Read the model definition and answer for the solid it produces. Units are mm, in the model's axes. Give positions to 0.01 mm unless a question says otherwise; leave off trailing zeros. Loops run counter-clockwise (first coordinate to the right, second up) from the corner with the lowest first, then second, coordinate; pieces in that order, holes last.
(1) Straight lines are drawn through the part: probe 1 along Y at (x, z) = (36.5, 6.25); probe 2 along Y at (x, z) = (0, 8.65); probe 3 along X at (y, z) = (-25, 2.2) (3 decimals). For each, find the intervals that lie inside material, in ascending order.
(2) Find section D-D, the plane z = 2.25. Write down the section's boundary in (x, y) (3 decimals), then the cut area to 3 significant figures.
(3) Find section B-B, the plane x = 0. Write down the section's boundary in (y, z) (3 decimals).
(4) This flat-tipped pin is pushed along its axis until it touches: P1, Ø3.5, axis at x = 2.5, y = 25, coming from the -Z side. Where does it stop, or does it pass through?
(5) Find section C-C, the plane y = -25. Write down the section's boundary in (x, z) (3 decimals).
(6) Find section A-A, the plane y = -36.5. Write down the section's boundary in (x, z), then the cut area to 3 significant figures.
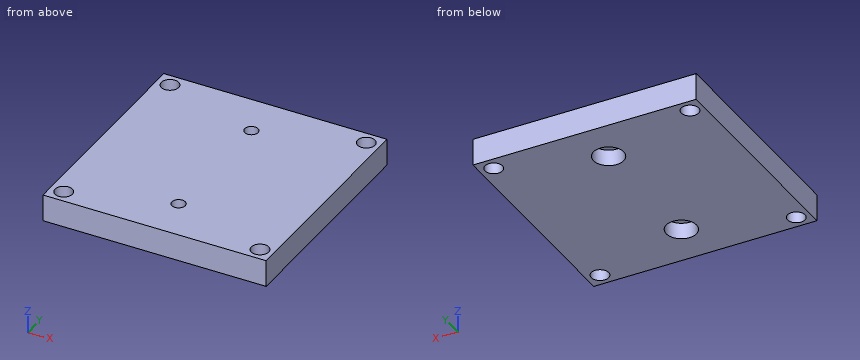
```python
from build123d import *

# Parameters (mm, degrees)
F0_W           = 83
F0_H           = 83
F1_DEPTH       = 10
F2_R           = 3.25
F3_DEPTH       = 10
F5_D           = 5
F5_DEPTH       = 15
F5_CBORE_D     = 11.25
F5_CBORE_DEPTH = 6
F5_TIP         = 1.5021515476


with BuildPart() as f1:
    # F0 (on Top) → F1 (new body)
    with BuildSketch(Plane.XY):
        Rectangle(F0_W, F0_H)
    extrude(amount=F1_DEPTH)

    # F2 (on face) → F3 (cut, through all)
    with BuildSketch(Plane.XY.offset(10)):
        with Locations((-36.5, 36.5)):
            Circle(F2_R)
        with Locations((-36.5, -36.5)):
            Circle(F2_R)
        with Locations((36.5, -36.5)):
            Circle(F2_R)
        with Locations((36.5, 36.5)):
            Circle(F2_R)
    extrude(amount=-F3_DEPTH, mode=Mode.SUBTRACT)

    # F5
    with Locations(Plane(origin=(0, 0, 0), x_dir=(1, 0, 0), z_dir=(0, 0, -1))):
        with Locations((0, -25), (0, 25)):
            CounterBoreHole(F5_D / 2, F5_CBORE_D / 2, F5_CBORE_DEPTH, depth=F5_DEPTH)
            with Locations((0, 0, -(F5_DEPTH + F5_TIP / 2))):  # 118° drill point
                Cone(0, F5_D / 2, F5_TIP, mode=Mode.SUBTRACT)


solid = f1.part
```
Entries:
1. probe 1: y = -41.5 to -39.75, -33.25 to 33.25, 39.75 to 41.5
1. probe 2: y = -41.5 to -27.5, -22.5 to 22.5, 27.5 to 41.5
1. probe 3: x = -41.5 to -5.625, 5.625 to 41.5
2. outline: (-41.5, -41.5) - (41.5, -41.5) - (41.5, 41.5) - (-41.5, 41.5) - close; hole circle Ø6.5 at (-36.5, -36.5); hole circle Ø6.5 at (-36.5, 36.5); hole circle Ø11.25 at (0, -25); hole circle Ø11.25 at (0, 25); hole circle Ø6.5 at (36.5, -36.5); hole circle Ø6.5 at (36.5, 36.5)
2. area: 6,560 mm2
3. outline: (-41.5, 0) - (-30.625, 0) - (-30.625, 6) - (-27.5, 6) - (-27.5, 10) - (-41.5, 10) - close; (-22.5, 6) - (-19.375, 6) - (-19.375, 0) - (19.375, 0) - (19.375, 6) - (22.5, 6) - (22.5, 10) - (-22.5, 10) - close; (27.5, 6) - (30.625, 6) - (30.625, 0) - (41.5, 0) - (41.5, 10) - (27.5, 10) - close
4. P1: stops at z = 6
5. outline: (-41.5, 0) - (-5.625, 0) - (-5.625, 6) - (-2.5, 6) - (-2.5, 10) - (-41.5, 10) - close; (2.5, 6) - (5.625, 6) - (5.625, 0) - (41.5, 0) - (41.5, 10) - (2.5, 10) - close
6. outline: (-41.5, 0) - (-39.75, 0) - (-39.75, 10) - (-41.5, 10) - close; (-33.25, 0) - (33.25, 0) - (33.25, 10) - (-33.25, 10) - close; (39.75, 0) - (41.5, 0) - (41.5, 10) - (39.75, 10) - close
6. area: 700 mm2
